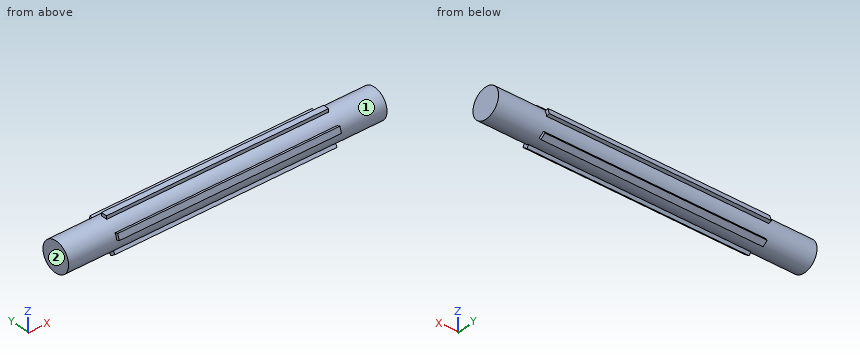
from build123d import *

# Parameters (mm, degrees)
SKETCH1_W           = 215
SKETCH1_H           = 10
SKETCH2_W           = 4
SKETCH2_H           = 4
BOSS_EXTRUDE1_DEPTH = 75
CIRPATTERN1_COUNT   = 5


with BuildPart() as part:
    # Sketch1 → Revolve1 (revolve)
    with BuildSketch(Plane.XY, mode=Mode.PRIVATE) as revolve1_sk:
        with Locations((0, 5)):
            Rectangle(SKETCH1_W, SKETCH1_H)
    revolve(revolve1_sk.sketch.rotate(Axis((0, 0, 0), (1, 0, 0)), 90), axis=Axis((0, 0, 0), (1, 0, 0)))

    # Sketch2 → Boss-Extrude1 (add, symmetric)
    with BuildSketch(Plane(origin=(0, 0, 0), x_dir=(0, 0, -1), z_dir=(1, 0, 0))):
        with Locations((-10, 0)):
            Rectangle(SKETCH2_W, SKETCH2_H)
    boss_extrude1 = extrude(amount=BOSS_EXTRUDE1_DEPTH, both=True)

    # CirPattern1: Boss-Extrude1 ×5 about axis
    cirpattern1_axis = Axis((0, 0, 0), (1, 0, 0))
    for i in range(1, CIRPATTERN1_COUNT):
        add(boss_extrude1.rotate(cirpattern1_axis, i * 360 / CIRPATTERN1_COUNT))


solid = part.part
Check sheet for the modelled part. Datum: model origin and axes. Units: mm. Face numbers are marked on the shaded views. Coordinates: 2 decimals unless noted, no trailing zeros. Loops run counter-clockwise (first coordinate to the right, second up) from the corner with the lowest first, then second, coordinate; pieces in that order, holes last. Notation, with made-up numbers: (42, -0.75) -> (85, -0.75) arc R24 ccw to (85, 34.25) -> close; hole circle Ø9 at (39, 68). An arc over 180 degrees is marked (long way). Answer in a Markdown table with one row per item.
1. Release check for a two-part mould opening along Y. For the marked faces 1 and 2 record: released by +Y, released by -Y, zero draft, split by the parting line, or undercut.
Check values:
| item | result |
|---|---|
| face 1 | undercut |
| face 2 | zero draft |
2. Go/stop test with flat-tipped pins: pin 1 (2.5 mm diameter, centred on x = 29.5, z = 10.5, fed in from -Y); pin 2 (4 mm diameter, centred on x = -48, z = 8, fed in from +Y); pin 3 (4 mm diameter, centred on x = -69.5, y = 7.5, fed in from -Z). Record where each tip stops, or that it passes through.
Check values:
| item | result |
|---|---|
| pin 1 | stops at y = -3.8 |
| pin 2 | stops at y = 8 |
| pin 3 | stops at z = -10.84 |
3. Sectioned sample at A-A, the plane y = 0. Record the boundary of the cut face in (x, z), then the cut area to 3 significant figures.
Check values:
| item | result |
|---|---|
| outline | (-107.5, -10) -> (107.5, -10) -> (107.5, 10) -> (75, 10) -> (75, 12) -> (-75, 12) -> (-75, 10) -> (-107.5, 10) -> close |
| area | 4,600 mm2 |
4. Sectioned sample at B-B, the plane x = 40. Record the boundary of the cut face in (y, z), then the cut area to 4 significant figures.
Check values:
| item | result |
|---|---|
| outline | (-12.03, 1.81) -> (-9.94, 1.13) arc R10 ccw to (-7.38, -6.75) -> (-8.67, -8.53) -> (-5.44, -10.88) -> (-4.14, -9.1) arc R10 ccw to (4.14, -9.1) -> (5.44, -10.88) -> (8.67, -8.53) -> (7.38, -6.75) arc R10 ccw to (9.94, 1.13) -> (12.03, 1.81) -> (10.79, 5.61) -> (8.7, 4.93) arc R10 ccw to (2, 9.8) -> (2, 12) -> (-2, 12) -> (-2, 9.8) arc R10 ccw to (-8.7, 4.93) -> (-10.79, 5.61) -> close |
| area | 355.5 mm2 |
5. Material ranges on line 1 along Z through (x, y) = (60, 0); line 2 along Y through (x, z) = (67, -8.5); line 3 along X through (y, z) = (-0.5, 10.5), recorded low to high. Write a range as [from, to].
Check values:
| item | result |
|---|---|
| line 1 | z = [-10, 12] |
| line 2 | y = [-8.65, 8.65] |
| line 3 | x = [-75, 75] |
